Part print with two shaded views. Sizes in mm from the minimum x, y, z corner. A direction names the side the tool comes from. Coordinates: 2 decimals unless noted, no trailing zeros. Loops run counter-clockwise (first coordinate to the right, second up) from the corner with the lowest first, then second, coordinate; pieces in that order, holes last. Notation, with made-up numbers: (6, 63.25) - (24, 63.25) arc R16 cw to (24, 74.25) - close; hole circle Ø10 at (50.5, 76.5). An arc over 180 degrees is marked (long way). Write each question's results on one line, items separated by ' | '. Start each with the question number.
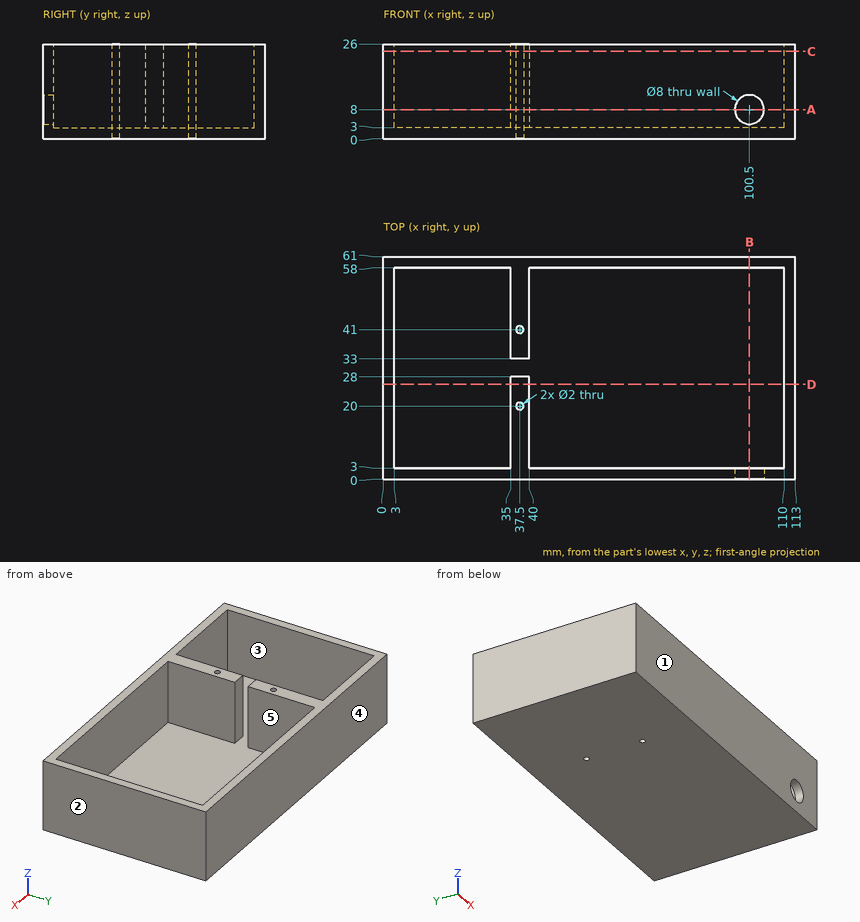
Q1. Cut at D-D (y = 26). List the corners of the cut face in (x, z), and give its area (3 significant figures).
Q2. Cut at B-B (x = 100.5). List the corners of the cut face in (y, z).
Q3. Which spindle directions (+Z, -Z, +X, -X, +Y, -Y) get a long thin tool onto all of the face, cutting with end or side? Do the marked faces 4 and 5. Say none if no direction does.
Q4. Cut at A-A (z = 8). List the corners of the cut face in (x, y).
Q5. Mould opens along Y. For the marked faces 1, 2 and 3 say: +Y half, -Y half, draft (parallel to the pull), parting line (faces both ways), or undercut.
Q6. Cut at C-C (z = 24). List the corners of the cut face in (x, y), and give its area (3 significant figures).
Q7. Drill centre lines: L1, parallel to X at y = 45, z = 11.5; L2, parallel to Y at x = 37.5, z = 9; L3, parallel to Y at x = 5, z = 20.5. Where is each one in solid material? Low to high. Write a range as from..to.
Check result:
1) outline: (0, 0) - (113, 0) - (113, 26) - (110, 26) - (110, 3) - (40, 3) - (40, 26) - (35, 26) - (35, 3) - (3, 3) - (3, 26) - (0, 26) - close | area: 592 mm²
2) outline: (0, 0) - (61, 0) - (61, 26) - (58, 26) - (58, 3) - (3, 3) - (3, 4) - (0, 4) - close; (0, 12) - (3, 12) - (3, 26) - (0, 26) - close
3) face 4: +Z, -Z, +X, -X, +Y | face 5: +Z
4) outline: (0, 0) - (96.5, 0) - (96.5, 3) - (40, 3) - (40, 28) - (35, 28) - (35, 3) - (3, 3) - (3, 58) - (35, 58) - (35, 33) - (40, 33) - (40, 58) - (110, 58) - (110, 3) - (104.5, 3) - (104.5, 0) - (113, 0) - (113, 61) - (0, 61) - close; hole circle Ø2 at (37.5, 20); hole circle Ø2 at (37.5, 41)
5) face 1: -Y half | face 2: draft | face 3: undercut
6) outline: (0, 0) - (113, 0) - (113, 61) - (0, 61) - close; hole (3, 3) - (35, 3) - (35, 28) - (40, 28) - (40, 3) - (110, 3) - (110, 58) - (40, 58) - (40, 33) - (35, 33) - (35, 58) - (3, 58) - close; hole circle Ø2 at (37.5, 20); hole circle Ø2 at (37.5, 41) | area: 1,250 mm²
7) L1: 0..3, 35..40, 110..113 | L2: 0..19, 21..28, 33..40, 42..61 | L3: 0..3, 58..61
